from build123d import *

# Parameters (mm, degrees)
SKETCH_1_W          = 20
SKETCH_1_H          = 20
SKETCH_1_W_2        = 16
SKETCH_1_H_2        = 16
EXTRUDE_1_DEPTH     = 560
SKETCH_4_R          = 2.2
CUT_EXTRUDE_3_DEPTH = 560
SKETCH_5_W          = 20
SKETCH_5_H          = 20
SKETCH_5_W_2        = 16
SKETCH_5_H_2        = 16
EXTRUDE_2_DEPTH     = 20
SKETCH_6_W          = 20
SKETCH_6_H          = 20
SKETCH_6_W_2        = 16
SKETCH_6_H_2        = 16
EXTRUDE_3_DEPTH     = 20
SKETCH_8_R          = 2.2
CUT_EXTRUDE_4_DEPTH = 20
SKETCH_9_R          = 2.2
CUT_EXTRUDE_5_DEPTH = 20
SKETCH_10_W         = 51.42245882
SKETCH_10_H         = 30.440795882
CUT_EXTRUDE_6_DEPTH = 40
SKETCH_11_W         = 39.362638682
SKETCH_11_H         = 52.74733359
CUT_EXTRUDE_7_DEPTH = 40
SKETCH_12_R         = 1
CUT_EXTRUDE_8_DEPTH = 10
SKETCH_13_R         = 1
CUT_EXTRUDE_9_DEPTH = 10
M4X0_7_1_D          = 3.3
M4X0_7_1_DEPTH      = 11.5
M4X0_7_1_TIP        = 0.991420021


with BuildPart() as part:
    # ｽｹｯﾁ1 → ﾎﾞｽ - 押し出し1 (new body)
    with BuildSketch(Plane.XY):
        Rectangle(SKETCH_1_W, SKETCH_1_H)
        Rectangle(SKETCH_1_W_2, SKETCH_1_H_2, mode=Mode.SUBTRACT)
    extrude(amount=EXTRUDE_1_DEPTH)

    # ｽｹｯﾁ4 → ｶｯﾄ - 押し出し3 (cut)
    with BuildSketch(Plane(origin=(0, 10, 0), x_dir=(1, 0, 0), z_dir=(0, 1, 0))):
        with Locations((0, -550)):
            Circle(SKETCH_4_R)
        with Locations((0, -10)):
            Circle(SKETCH_4_R)
    extrude(amount=-CUT_EXTRUDE_3_DEPTH, mode=Mode.SUBTRACT)

    # ｽｹｯﾁ5 → ﾎﾞｽ - 押し出し2 (add)
    with BuildSketch(Plane(origin=(0, 0, 0), x_dir=(-1, 0, 0), z_dir=(0, 0, -1))):
        Rectangle(SKETCH_5_W, SKETCH_5_H)
        Rectangle(SKETCH_5_W_2, SKETCH_5_H_2, mode=Mode.SUBTRACT)
    extrude(amount=EXTRUDE_2_DEPTH)

    # ｽｹｯﾁ6 → ﾎﾞｽ - 押し出し3 (add)
    with BuildSketch(Plane.XY.offset(560)):
        Rectangle(SKETCH_6_W, SKETCH_6_H)
        Rectangle(SKETCH_6_W_2, SKETCH_6_H_2, mode=Mode.SUBTRACT)
    extrude(amount=EXTRUDE_3_DEPTH)

    # ｽｹｯﾁ8 → ｶｯﾄ - 押し出し4 (cut)
    with BuildSketch(Plane(origin=(10, 0, 0), x_dir=(0, 0, -1), z_dir=(1, 0, 0))):
        with Locations((-570, 0)):
            Circle(SKETCH_8_R)
    extrude(amount=-CUT_EXTRUDE_4_DEPTH, mode=Mode.SUBTRACT)

    # ｽｹｯﾁ9 → ｶｯﾄ - 押し出し5 (cut)
    with BuildSketch(Plane(origin=(10, 0, 0), x_dir=(0, 0, -1), z_dir=(1, 0, 0))):
        with Locations((10, 0)):
            Circle(SKETCH_9_R)
    extrude(amount=-CUT_EXTRUDE_5_DEPTH, mode=Mode.SUBTRACT)

    # ｽｹｯﾁ10 → ｶｯﾄ - 押し出し6 (cut)
    with BuildSketch(Plane(origin=(0, 0, -20), x_dir=(-1, 0, 0), z_dir=(0, 0, -1))):
        Rectangle(SKETCH_10_W, SKETCH_10_H)
    extrude(amount=-CUT_EXTRUDE_6_DEPTH, mode=Mode.SUBTRACT)

    # ｽｹｯﾁ11 → ｶｯﾄ - 押し出し7 (cut)
    with BuildSketch(Plane.XY.offset(580)):
        Rectangle(SKETCH_11_W, SKETCH_11_H)
    extrude(amount=-CUT_EXTRUDE_7_DEPTH, mode=Mode.SUBTRACT)

    # ｽｹｯﾁ12 → ｶｯﾄ - 押し出し8 (cut)
    with BuildSketch(Plane(origin=(0, -10, 0), x_dir=(-1, 0, 0), z_dir=(0, -1, 0))):
        with Locations((0, -530)):
            Circle(SKETCH_12_R)
        with Locations((0, -510)):
            Circle(SKETCH_12_R)
    extrude(amount=-CUT_EXTRUDE_8_DEPTH, mode=Mode.SUBTRACT)

    # ｽｹｯﾁ13 → ｶｯﾄ - 押し出し9 (cut)
    with BuildSketch(Plane(origin=(0, -10, 0), x_dir=(-1, 0, 0), z_dir=(0, -1, 0))):
        with Locations((0, -30)):
            Circle(SKETCH_13_R)
        with Locations((0, -50)):
            Circle(SKETCH_13_R)
    extrude(amount=-CUT_EXTRUDE_9_DEPTH, mode=Mode.SUBTRACT)

    # M4x0.7 ねじ穴1
    with Locations(Plane(origin=(0, -10, 30), x_dir=(0, 0, -1), z_dir=(0, -1, 0))):
        with Locations((0, 0), (-20, 0), (-480, 0), (-500, 0)):
            Hole(M4X0_7_1_D / 2, depth=M4X0_7_1_DEPTH)
            with Locations((0, 0, -(M4X0_7_1_DEPTH + M4X0_7_1_TIP / 2))):  # 118° drill point
                Cone(0, M4X0_7_1_D / 2, M4X0_7_1_TIP, mode=Mode.SUBTRACT)


solid = part.part
Geometry check sheet. Reference: the model listing, model coordinates, mm. A direction names the side the tool comes from. Give positions to 0.01 mm unless a question says otherwise; leave off trailing zeros. Order: outer loops, then holes, each group sorted by start corner. A loop starts at its lowest first (then second) coordinate and runs counter-clockwise, first axis right, second up. Notation, with made-up numbers: (32, -1.5) - (67, -1.5) arc R20 cw to (67, 27.5) - close; hole circle Ø3 at (40.25, 22.25). An arc over 180 degrees is marked (long way). Answer as a JSON object with one key per item and string values.
(1) Tool access check on faces 1 (the flat face through (0, -8, 276)), 2 (the flat face through (0, -10, 276)). Record the directions out of +Z, -Z, +X, -X, +Y, -Y that give a thin tool (end or side, any length) a straight path to the whole face; none if there is none.
Report:
{"face 1": "+Z, -Z", "face 2": "+Z, -Z, +X, -X, -Y"}
(2) Draft check along X on faces 3 (the flat face through (9, 0, 20)), 4 (the flat face through (-10, 0, 276)), 5 (the flat face through (8, 0, 276)). Enter one of: released by +X, released by -X, zero draft, split by the parting line, or undercut.
Report:
{"face 3": "zero draft", "face 4": "released by -X", "face 5": "undercut"}
(3) Material ranges on line 1 (X direction, y = -0.75, z = 474); line 2 (X direction, y = -8.45, z = 30), recorded low to high.
Report:
{"line 1": "-10 to -8, 8 to 10", "line 2": "-10 to -1.65, 1.65 to 10"}
(4) Cross-section at B-B (z = 344.5). Record the cut outline in (x, y).
Report:
{"outline": "(-10, -10) - (10, -10) - (10, 10) - (-10, 10) - close; hole (-8, -8) - (8, -8) - (8, 8) - (-8, 8) - close"}
(5) Cross-section at A-A (y = -3.5). Record the cut outline in (x, z), then the cut area to 3 significant figures.
Report:
{"outline": "(-10, 20) - (-8, 20) - (-8, 540) - (-10, 540) - close; (8, 20) - (10, 20) - (10, 540) - (8, 540) - close", "area": "2,080 mm^2"}
(6) Depth check by flat-ended pin: pin 1 Ø2.5 at (x, z) = (0, 30) entering from -Y. Enter the tip coordinate at first touch or a pass-through.
Report:
{"pin 1": "y = 8"}
